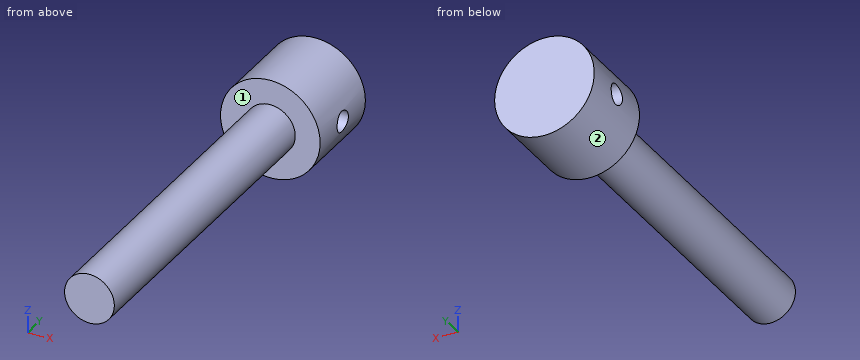
from build123d import *

# Parameters (mm, degrees)
SKETCH1_R               = 152.4
BOSS_EXTRUDE1_DEPTH     = 2540
SKETCH1_3_R             = 304.8
SKETCH1_3_R_2           = 152.4
BOSS_EXTRUDE2_DEPTH     = 508
SKETCH2_R               = 63.5
CUT_EXTRUDE1_DEPTH      = 305.8
CUT_EXTRUDE1_DEPTH_BACK = 305.8


with BuildPart() as part:
    # Sketch1 → Boss-Extrude1 (new body)
    with BuildSketch(Plane(origin=(0, 0, 0), x_dir=(1, 0, 0), z_dir=(0, 1, 0))):
        Circle(SKETCH1_R)
    extrude(amount=-BOSS_EXTRUDE1_DEPTH)

    # Sketch1<3> → Boss-Extrude2 (add)
    with BuildSketch(Plane(origin=(0, 0, 0), x_dir=(1, 0, 0), z_dir=(0, 1, 0))):
        Circle(SKETCH1_3_R)
        Circle(SKETCH1_3_R_2, mode=Mode.SUBTRACT)
    extrude(amount=-BOSS_EXTRUDE2_DEPTH)

    # Sketch2 → Cut-Extrude1 (cut, two sides)
    with BuildSketch(Plane(origin=(0, 0, 0), x_dir=(0, 0, -1), z_dir=(1, 0, 0))) as cut_extrude1_sk:
        with Locations((0, -254)):
            Circle(SKETCH2_R)
    extrude(amount=CUT_EXTRUDE1_DEPTH, mode=Mode.SUBTRACT)
    extrude(cut_extrude1_sk.sketch, amount=-CUT_EXTRUDE1_DEPTH_BACK, mode=Mode.SUBTRACT)


solid = part.part
Could you check a few things on this model? Use its own coordinates, in mm. Face numbers are marked on the shaded views. A direction names the side the tool comes from. Give positions to 0.01 mm unless a question says otherwise; leave off trailing zeros. Order: outer loops, then holes, each group sorted by start corner. A loop starts at its lowest first (then second) coordinate and runs counter-clockwise, first axis right, second up. Notation, with made-up numbers: (-31.5, 53) - (-16.5, 53) arc R8 ccw to (-16.5, 68) - close; hole circle Ø10 at (38.25, -5). An arc over 180 degrees is marked (long way). Return JSON: item names as keys, results as strings. Group by question number.
Q1. Please list where these lines run through material, in increasing order: line 1 along Y through (x, z) = (202, 0); line 2 along Y through (x, z) = (-181.5, 233); line 3 along Y through (x, z) = (-62.5, 0). Write a range as [from, to].
Q2. Suppose I cut it at D-D, the plane z = -98.5. Please give me the cut outline in (x, y).
Q3. Which directions (+Z, -Z, +X, -X, +Y, -Y) give clear straight access to the entire face, cutting with the end or side of a thin tool? Please do the marked faces 1 and 2.
Q4. Suppose I cut it at B-B, the plane x = 25. Please give me the cut outline in (y, z).
Q5. Will these pins go through, and if not, where does the flat tip stop? pin 1 Ø1.5 at (x, z) = (6, -185) entering from -Y; pin 2 Ø4 at (x, y) = (-102, -1996) entering from +Z; pin 3 Ø5 at (y, z) = (-454, 203.5) entering from +X.
Q6. Suppose I cut it at A-A, the plane z = 0. Please give me the cut outline in (x, y).
Q7. Suppose I cut it at C-C, the plane y = -810. Please give me the cut outline in (x, z).
Resolved:
{
 "1": {"line 1": "y = [-508, -317.5], [-190.5, 0]", "line 2": "y = [-508, 0]", "line 3": "y = [-2540, -317.5], [-190.5, 0]"},
 "2": {"outline": "(-288.45, -508) - (-116.29, -508) - (-116.29, -2540) - (116.29, -2540) - (116.29, -508) - (288.45, -508) - (288.45, 0) - (-288.45, 0) - close"},
 "3": {"face 1": "-Y", "face 2": "+Y, -Y"},
 "4": {"outline": "(-2540, -150.34) - (-508, -150.34) - (-508, -303.77) - (0, -303.77) - (0, 303.77) - (-508, 303.77) - (-508, 150.34) - (-2540, 150.34) - close; hole circle Ø127 at (-254, 0)"},
 "5": {"pin 1": "stops at y = -508", "pin 2": "stops at z = 115", "pin 3": "stops at x = 229.13"},
 "6": {"outline": "(-304.8, -508) - (-152.4, -508) - (-152.4, -2540) - (152.4, -2540) - (152.4, -508) - (304.8, -508) - (304.8, -317.5) - (-304.8, -317.5) - close; (-304.8, -190.5) - (304.8, -190.5) - (304.8, 0) - (-304.8, 0) - close"},
 "7": {"outline": "circle Ø304.8 at (0, 0)"}
}
